Could you check a few things on this model? Use its own coordinates, in mm. A direction names the side the tool comes from. Coordinates: 2 decimals unless noted, no trailing zeros. Order: outer loops, then holes, each group sorted by start corner. A loop starts at its lowest first (then second) coordinate and runs counter-clockwise, first axis right, second up. Notation, with made-up numbers: (39, 82) - (84, 82) arc R26 ccw to (84, 100) - close; hole circle Ø6 at (-2, 71). An arc over 180 degrees is marked (long way). Answer as a JSON object with one key per item and string values. Group by question number.
(1) Which directions (+Z, -Z, +X, -X, +Y, -Y) give clear straight access to the entire face, cutting with the end or side of a thin tool? Please do faces 4 (the flat face through (-19.05, 0, -39)), 5 (the cylindrical face through (-8.972, -0.133, -45.133)).
(2) Imagine slicing it at D-D, the plane x = -28. Write out the boundary of the cut face in (y, z) (3 decimals), and give its area (3 significant figures).
(3) Imagine slicing it at C-C, the plane x = -9. Write out the boundary of the cut face in (y, z) (3 decimals), and give its area (3 significant figures).
(4) We'd pull the mould along Z, two halves only. Please class faces 1 (the cylindrical face through (-9.193, -0.133, -31.106)), 2 (the flat face through (-15, -9.525, -23)), 3 (the flat face through (-38, 0, -19.05)): pulls with the +Z half, pulls with the -Z half, needs draft (parallel to the pull), parting line crosses it, or undercut.
(5) Imagine slicing it at B-B, the plane y = 1.5. Write out the boundary of the cut face in (x, z) (3 decimals), and give its area (3 significant figures).
(6) Will these pins go through, and if not, where does the flat tip stop? P1, Ø1.5, axis at x = -37.5, y = -6.5, coming from the -Z side; P2, Ø4.5, axis at x = -47.625, z = -9.525, coming from the -Y side; P3, Ø6, axis at y = 3, z = -48.5, coming from the -X side.
(7) Imagine slicing it at A-A, the plane z = -46.5. Write out the boundary of the cut face in (x, y) (3 decimals).
(8) Please list where these lines run through material, in increasing order: probe 1 along Z at (x, y) = (-47.5, -8); probe 2 along X at (y, z) = (-6.75, -9); probe 3 along X at (y, z) = (-0.25, -42.5).
Autodesk Inventor part; units mm, degrees
ref_plane "YZ Plane" through (0, 0, 0) normal (1, 0, 0) x (0, 1, 0)
ref_plane "XZ Plane" through (0, 0, 0) normal (0, 1, 0) x (-1, 0, 0)
ref_plane "XY Plane" through (0, 0, 0) normal (0, 0, 1) x (1, 0, 0)
sketch "Sketch1" plane through (0, 0, 0) normal (0, 1, 0) x (-1, 0, 0)
  line L0 (0, 0) -> (57.15, 0)
  line L1 (57.15, 0) -> (57.15, -19.05)
  line L2 (57.15, -19.05) -> (19.05, -19.05)
  line L3 (19.05, -19.05) -> (19.05, -59.69)
  line L4 (19.05, -59.69) -> (0, -59.69)
  line L5 (0, -59.69) -> (0, 0)
  circle A0 centre (28.575, -9.525) radius 2.5527
  circle A1 centre (47.625, -9.525) radius 2.5527
  line L6 (19.05, -19.05) -> (0, 0) construction
  circle A2 centre (9.525, -28.575) radius 2.5527
  circle A3 centre (9.525, -47.625) radius 2.5527
  circle A4 centre (9.525, -9.525) radius 2.5527
  point P0 (57.15, -9.525)
  dimension "d0" = 19.05
  dimension "d1" = 19.05
  dimension "d2" = 59.69
  dimension "d3" = 57.15
  dimension "d4" = 5.1054
  dimension "d5" = 28.575
  dimension "d6" = 19.05
extrude "Extrusion1" add sketch "Sketch1" along normal mid plane 19.05
thread "Thread1"
thread "Thread2"
thread "Thread3"
thread "Thread4"
thread "Thread5"
properties part number "STRU_025_DoubleBillet_90_2.25in_2" material "Aluminum 6061"
Result set:
{
 "1": {"face 4": "-Z, -X, +Y, -Y", "face 5": "+Y, -Y"},
 "2": {"outline": "(-9.525, -19.05) - (9.525, -19.05) - (9.525, -12.012) - (-9.525, -12.012) - close; (-9.525, -7.038) - (9.525, -7.038) - (9.525, 0) - (-9.525, 0) - close", "area": "268 mm^2"},
 "3": {"outline": "(-9.525, -59.69) - (9.525, -59.69) - (9.525, -50.123) - (-9.525, -50.123) - close; (-9.525, -45.127) - (9.525, -45.127) - (9.525, -31.073) - (-9.525, -31.073) - close; (-9.525, -26.077) - (9.525, -26.077) - (9.525, -12.023) - (-9.525, -12.023) - close; (-9.525, -7.027) - (9.525, -7.027) - (9.525, 0) - (-9.525, 0) - close", "area": "852 mm^2"},
 "4": {"face 1": "undercut", "face 2": "needs draft", "face 3": "pulls with the -Z half"},
 "5": {"outline": "(-57.15, -19.05) - (-19.05, -19.05) - (-19.05, -59.69) - (0, -59.69) - (0, 0) - (-57.15, 0) - close; hole circle Ø5.105 at (-47.625, -9.525); hole circle Ø5.105 at (-28.575, -9.525); hole circle Ø5.105 at (-9.525, -47.625); hole circle Ø5.105 at (-9.525, -28.575); hole circle Ø5.105 at (-9.525, -9.525)", "area": "1,760 mm^2"},
 "6": {"P1": "stops at z = -19.05", "P2": "passes through", "P3": "stops at x = -19.05"},
 "7": {"outline": "(-19.05, -9.525) - (-11.816, -9.525) - (-11.816, 9.525) - (-19.05, 9.525) - close; (-7.234, -9.525) - (0, -9.525) - (0, 9.525) - (-7.234, 9.525) - close"},
 "8": {"probe 1": "z = -19.05 to -12.07, -6.98 to 0", "probe 2": "x = -57.15 to -50.12, -45.13 to -31.07, -26.08 to -12.02, -7.03 to 0", "probe 3": "x = -19.05 to 0"}
}
